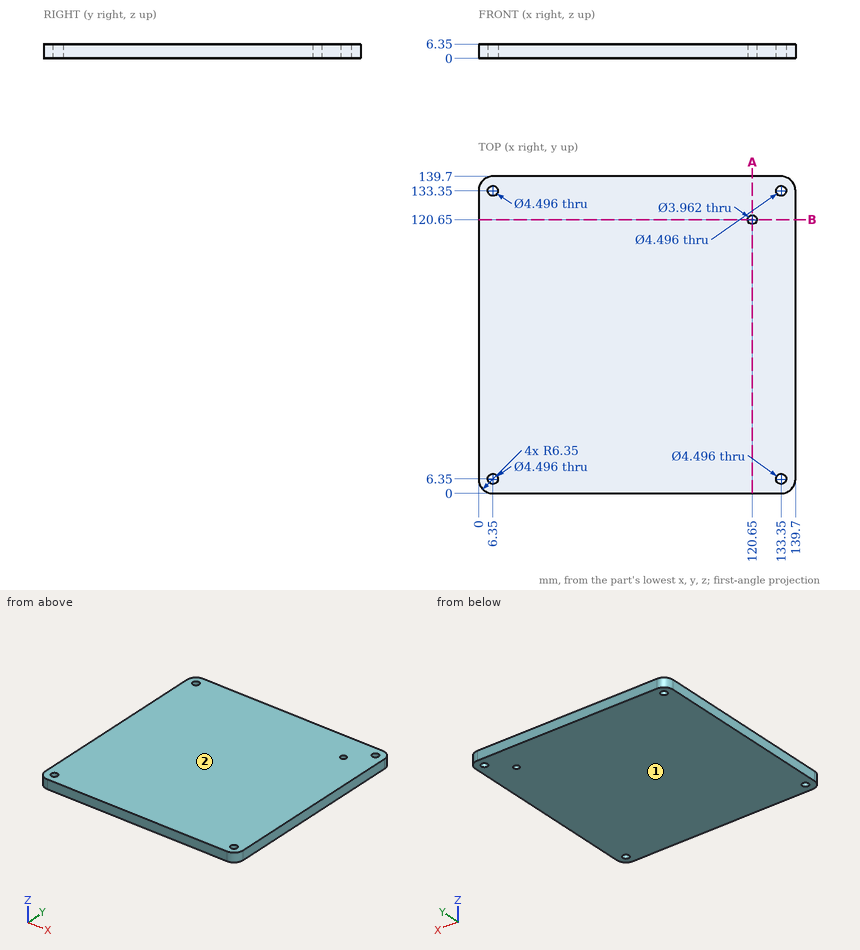
Here's the drawing with two shaded views (mm, measured from the low corner). I have some questions. Give positions to 0.01 mm unless a question says otherwise; leave off trailing zeros. Write each loop counter-clockwise with the first axis right and the second up, starting at its lowest first coordinate (ties: lowest second). Pieces come first, ordered by that corner, then holes. Notation, with made-up numbers: (-1.5, 72.25) -> (9.5, 72.25) arc R37 cw to (9.5, 109.25) -> close; hole circle Ø1 at (3.25, -9.5). An arc over 180 degrees is marked (long way). Answer as a JSON object with one key per item and string values. Group by question number.
Item 1: Suppose I cut it at A-A (x = 120.65). Please give me the cut outline in (y, z), plus the area to 3 significant figures.
Item 2: I'm going to push a flat-ended pin straight in: P1, Ø3, axis at x = 120.65, y = 120.65, coming from the -Z side. Where does the tip first touch, or does it pass through?
Item 3: Please list where these lines run through material, in increasing order: line 1 (X direction, y = 6.35, z = 2.5); line 2 (X direction, y = 120.65, z = 2.75). Write a range as [from, to].
Item 4: We'd pull the mould along Z, two halves only. Please class the marked faces 1 and 2: +Z half, -Z half, draft (parallel to the pull), parting line (faces both ways), or undercut.
Findings:
{
 "1": {"outline": "(0, 0) -> (118.67, 0) -> (118.67, 6.35) -> (0, 6.35) -> close; (122.63, 0) -> (139.7, 0) -> (139.7, 6.35) -> (122.63, 6.35) -> close", "area": "862 mm²"},
 "2": {"P1": "passes through"},
 "3": {"line 1": "x = [0, 4.1], [8.6, 131.1], [135.6, 139.7]", "line 2": "x = [0, 118.67], [122.63, 139.7]"},
 "4": {"face 1": "-Z half", "face 2": "+Z half"}
}
